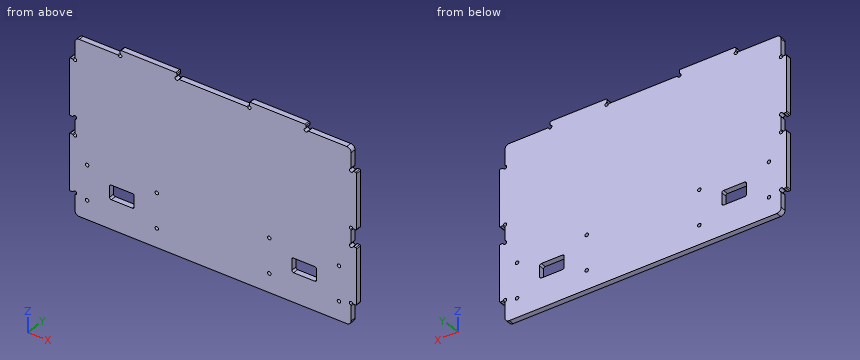
from build123d import *

# Parameters (mm, degrees)
SKETCH1_W              = 317.3
SKETCH1_H              = 363.32
BOSS_EXTRUDE1_DEPTH    = 6.35
SKETCH11_W             = 28.32
SKETCH11_H             = 16.5
CUT_EXTRUDE8_DEPTH     = 7.35
SKETCH12_R             = 2
CUT_EXTRUDE9_DEPTH     = 7.35
FILLET4_R              = 2
SKETCH14_W             = 317.3
SKETCH14_H             = 163.32
CUT_EXTRUDE10_DEPTH    = 6.35
SKETCH15_W             = 6.35
SKETCH15_H             = 65
BOSS_EXTRUDE2_DEPTH    = 6.35
SKETCH16_R             = 2
CUT_EXTRUDE11_DEPTH    = 6.35
FILLET5_R              = 1
LPATTERN1_COUNT        = 2
LPATTERN1_PITCH        = 85
FILLET5_OF_LPATTERN1_R = 1
FILLET6_R              = 5
SKETCH18_W             = 6.35
SKETCH18_H             = 65
BOSS_EXTRUDE3_DEPTH    = 6.35
SKETCH19_R             = 2
CUT_EXTRUDE12_DEPTH    = 6.35
FILLET7_R              = 1
LPATTERN2_COUNT        = 2
LPATTERN2_PITCH        = 85
FILLET7_OF_LPATTERN2_R = 1
SKETCH20_W             = 65
SKETCH20_H             = 6.35
BOSS_EXTRUDE4_DEPTH    = 6.35
SKETCH21_R             = 2
CUT_EXTRUDE13_DEPTH    = 6.35
FILLET8_R              = 1
FILLET8_OF_MIRROR10_R  = 1


with BuildPart() as part:
    # Sketch1 → Boss-Extrude1 (new body)
    with BuildSketch(Plane(origin=(0, 0, 0), x_dir=(1, 0, 0), z_dir=(0, 1, 0))):
        Rectangle(SKETCH1_W, SKETCH1_H)
    extrude(amount=-BOSS_EXTRUDE1_DEPTH)

    # Sketch11 → Cut-Extrude8 (cut, through all)
    with BuildSketch(Plane(origin=(0, 0, 0), x_dir=(1, 0, 0), z_dir=(0, 1, 0))):
        with Locations((104.666666667, -23.41)):
            Rectangle(SKETCH11_W, SKETCH11_H)
    cut_extrude8 = extrude(amount=-CUT_EXTRUDE8_DEPTH, mode=Mode.SUBTRACT)

    # Sketch12 → Cut-Extrude9 (cut, through all)
    with BuildSketch(Plane(origin=(0, 0, 0), x_dir=(1, 0, 0), z_dir=(0, 1, 0))):
        with Locations((64.666666667, -3.41)):
            Circle(SKETCH12_R)
        with Locations((144.666666667, -3.41)):
            Circle(SKETCH12_R)
        with Locations((144.666666667, -43.41)):
            Circle(SKETCH12_R)
        with Locations((64.666666667, -43.41)):
            Circle(SKETCH12_R)
    cut_extrude9 = extrude(amount=-CUT_EXTRUDE9_DEPTH, mode=Mode.SUBTRACT)

    # Mirror3: Cut-Extrude8, Cut-Extrude9 across plane
    add(cut_extrude8.mirror(Plane(origin=(0, 0, 0), x_dir=(0, 0, 1), z_dir=(1, 0, 0))), mode=Mode.SUBTRACT)
    add(cut_extrude9.mirror(Plane(origin=(0, 0, 0), x_dir=(0, 0, 1), z_dir=(1, 0, 0))), mode=Mode.SUBTRACT)

    # Fillet4
    fillet4_edges = [part.edges().sort_by_distance(p)[0] for p in [
        (90.506666667, -3.175, 31.66),
        (90.506666667, -3.175, 15.16),
        (118.826666667, -3.175, 15.16),
        (118.826666667, -3.175, 31.66),
        (-90.506666667, -3.175, 15.16),
        (-90.506666667, -3.175, 31.66),
        (-118.826666667, -3.175, 31.66),
        (-118.826666667, -3.175, 15.16),
    ]]
    fillet(fillet4_edges, radius=FILLET4_R)

    # Sketch14 → Cut-Extrude10 (cut)
    with BuildSketch(Plane(origin=(0, 0, 0), x_dir=(1, 0, 0), z_dir=(0, 1, 0))):
        with Locations((0, 100)):
            Rectangle(SKETCH14_W, SKETCH14_H)
    extrude(amount=-CUT_EXTRUDE10_DEPTH, mode=Mode.SUBTRACT)

    # Sketch15 → Boss-Extrude2 (add)
    with BuildSketch(Plane(origin=(0, 0, 0), x_dir=(1, 0, 0), z_dir=(0, 1, 0))):
        with Locations((161.825, -39.16)):
            Rectangle(SKETCH15_W, SKETCH15_H)
    boss_extrude2 = extrude(amount=-BOSS_EXTRUDE2_DEPTH)

    # Sketch16 → Cut-Extrude11 (cut)
    with BuildSketch(Plane(origin=(0, 0, 0), x_dir=(1, 0, 0), z_dir=(0, 1, 0))):
        with Locations((158.65, -71.66)):
            Circle(SKETCH16_R)
        with Locations((158.65, -6.66)):
            Circle(SKETCH16_R)
    cut_extrude11 = extrude(amount=-CUT_EXTRUDE11_DEPTH, mode=Mode.SUBTRACT)

    # Fillet5
    fillet5_edges = [part.edges().sort_by_distance(p)[0] for p in [
        (165, -3.175, 6.66),
        (165, -3.175, 71.66),
        (160.65, -3.175, 71.66),
        (160.65, -3.175, 6.66),
        (158.65, -3.175, 73.66),
        (158.65, -3.175, 4.66),
    ]]
    fillet(fillet5_edges, radius=FILLET5_R)

    # LPattern1: Boss-Extrude2, Cut-Extrude11 ×2
    with Locations(*[(0, 0, i * LPATTERN1_PITCH) for i in range(1, LPATTERN1_COUNT)]):
        add(boss_extrude2)
        add(cut_extrude11, mode=Mode.SUBTRACT)

    # Fillet5 of LPattern1
    fillet5_of_lpattern1_edges = [part.edges().sort_by_distance(p)[0] for p in [
        (165, -3.175, 91.66),
        (165, -3.175, 156.66),
        (160.65, -3.175, 156.66),
        (160.65, -3.175, 91.66),
        (158.65, -3.175, 158.66),
        (158.65, -3.175, 89.66),
    ]]
    fillet(fillet5_of_lpattern1_edges, radius=FILLET5_OF_LPATTERN1_R)

    # Fillet6
    fillet6_edges = [part.edges().sort_by_distance(p)[0] for p in [
        (158.65, -3.175, -18.34),
        (-158.65, -3.175, -18.34),
        (158.65, -3.175, 181.66),
        (-158.65, -3.175, 181.66),
    ]]
    fillet(fillet6_edges, radius=FILLET6_R)

    # Sketch18 → Boss-Extrude3 (add)
    with BuildSketch(Plane(origin=(0, 0, 0), x_dir=(1, 0, 0), z_dir=(0, 1, 0))):
        with Locations((-161.825, -39.16)):
            Rectangle(SKETCH18_W, SKETCH18_H)
    boss_extrude3 = extrude(amount=-BOSS_EXTRUDE3_DEPTH)

    # Sketch19 → Cut-Extrude12 (cut)
    with BuildSketch(Plane(origin=(0, 0, 0), x_dir=(1, 0, 0), z_dir=(0, 1, 0))):
        with Locations((-158.65, -6.66)):
            Circle(SKETCH19_R)
        with Locations((-158.65, -71.66)):
            Circle(SKETCH19_R)
    cut_extrude12 = extrude(amount=-CUT_EXTRUDE12_DEPTH, mode=Mode.SUBTRACT)

    # Fillet7
    fillet7_edges = [part.edges().sort_by_distance(p)[0] for p in [
        (-165, -3.175, 71.66),
        (-165, -3.175, 6.66),
        (-160.65, -3.175, 6.66),
        (-160.65, -3.175, 71.66),
        (-158.65, -3.175, 4.66),
        (-158.65, -3.175, 73.66),
    ]]
    fillet(fillet7_edges, radius=FILLET7_R)

    # LPattern2: Boss-Extrude3, Cut-Extrude12 ×2
    with Locations(*[(0, 0, i * LPATTERN2_PITCH) for i in range(1, LPATTERN2_COUNT)]):
        add(boss_extrude3)
        add(cut_extrude12, mode=Mode.SUBTRACT)

    # Fillet7 of LPattern2
    fillet7_of_lpattern2_edges = [part.edges().sort_by_distance(p)[0] for p in [
        (-165, -3.175, 156.66),
        (-165, -3.175, 91.66),
        (-160.65, -3.175, 91.66),
        (-160.65, -3.175, 156.66),
        (-158.65, -3.175, 89.66),
        (-158.65, -3.175, 158.66),
    ]]
    fillet(fillet7_of_lpattern2_edges, radius=FILLET7_OF_LPATTERN2_R)

    # Sketch20 → Boss-Extrude4 (add)
    with BuildSketch(Plane(origin=(0, 0, 0), x_dir=(1, 0, 0), z_dir=(0, 1, 0))):
        with Locations((74.15, -184.835)):
            Rectangle(SKETCH20_W, SKETCH20_H)
    boss_extrude4 = extrude(amount=-BOSS_EXTRUDE4_DEPTH)

    # Sketch21 → Cut-Extrude13 (cut)
    with BuildSketch(Plane(origin=(0, 0, 0), x_dir=(1, 0, 0), z_dir=(0, 1, 0))):
        with Locations((41.65, -181.66)):
            Circle(SKETCH21_R)
        with Locations((106.65, -181.66)):
            Circle(SKETCH21_R)
    cut_extrude13 = extrude(amount=-CUT_EXTRUDE13_DEPTH, mode=Mode.SUBTRACT)

    # Fillet8
    fillet8_edges = [part.edges().sort_by_distance(p)[0] for p in [
        (41.65, -3.175, 188.01),
        (106.65, -3.175, 188.01),
        (106.65, -3.175, 183.66),
        (41.65, -3.175, 183.66),
        (39.65, -3.175, 181.66),
        (108.65, -3.175, 181.66),
    ]]
    fillet(fillet8_edges, radius=FILLET8_R)

    # Mirror10: Boss-Extrude4, Cut-Extrude13 across plane
    add(boss_extrude4.mirror(Plane(origin=(0, 0, 0), x_dir=(0, 0, 1), z_dir=(1, 0, 0))))
    add(cut_extrude13.mirror(Plane(origin=(0, 0, 0), x_dir=(0, 0, 1), z_dir=(1, 0, 0))), mode=Mode.SUBTRACT)

    # Fillet8 of Mirror10
    fillet8_of_mirror10_edges = [part.edges().sort_by_distance(p)[0] for p in [
        (-41.65, -3.175, 188.01),
        (-106.65, -3.175, 188.01),
        (-106.65, -3.175, 183.66),
        (-41.65, -3.175, 183.66),
        (-39.65, -3.175, 181.66),
        (-108.65, -3.175, 181.66),
    ]]
    fillet(fillet8_of_mirror10_edges, radius=FILLET8_OF_MIRROR10_R)


solid = part.part
The model under review builds one solid part; all positions refer to its coordinate system, in mm. Round coordinates to 2 decimals unless told otherwise and drop trailing zeros. Loops run counter-clockwise (first coordinate to the right, second up) from the corner with the lowest first, then second, coordinate; pieces in that order, holes last. Notation, with made-up numbers: (85.5, 43) -> (108.5, 43) arc R27 cw to (108.5, 62) -> close; hole circle Ø9 at (49, 4.5). An arc over 180 degrees is marked (long way). Return JSON: item names as keys, results as strings.
(1) For line 1 (X direction, y = -1.5, z = 27); line 2 (Z direction, x = -144.5, y = -0.75); line 3 (X direction, y = -2.5, z = 3.41), list the stretches that pass through material, from the lowest coordinate up.
Solved:
{"line 1": "-165 to -118.83, -90.51 to 90.51, 118.83 to 165", "line 2": "-18.34 to 1.42, 5.4 to 41.42, 45.4 to 181.66", "line 3": "-158.65 to -146.67, -142.67 to -66.67, -62.67 to 62.67, 66.67 to 142.67, 146.67 to 158.65"}
(2) Add section C-C on z = 173. Write out the cut boundary in (x, y), plus the area to 3 significant figures.
Solved:
{"outline": "(-158.65, -6.35) -> (158.65, -6.35) -> (158.65, 0) -> (-158.65, 0) -> close", "area": "2,010 mm2"}
(3) Add section A-A on y = -1.5. State how many separate pieces and enclosed holes the cut face has, plus the area to 3 significant figures.
Solved:
{"separate pieces": "1", "enclosed holes": "10", "area": "64,800 mm2"}
(4) Add section B-B on x = -122.5. Write out the cut boundary in (y, z), plus the area to 3 significant figures.
Solved:
{"outline": "(-6.35, -18.34) -> (0, -18.34) -> (0, 181.66) -> (-6.35, 181.66) -> close", "area": "1,270 mm2"}
(5) For pin 1 (0.8 mm diameter, centred on x = -163, y = -2.5, fed in from -Z); pin 2 (1.3 mm diameter, centred on y = -3, z = 186, fed in from +X); pin 3 (3 mm diameter, centred on x = 134, y = -3, fed in from +Z), all flat-tipped, find the tip position at first contact; note any pin that passes through.
Solved:
{"pin 1": "z = 6.66", "pin 2": "x = 106.65", "pin 3": "z = 181.66"}
